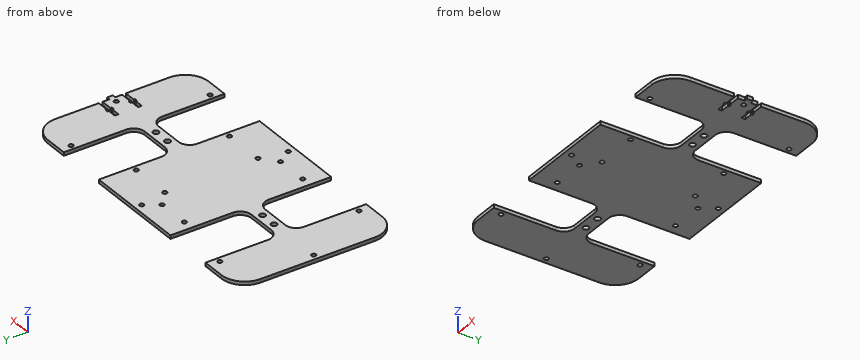
```python
from build123d import *

# Parameters (mm, degrees)
PAD_DEPTH       = 3
SKETCH004_R     = 2.5
POCKET_DEPTH    = 588.208656
SKETCH005_R     = 1.9
POCKET001_DEPTH = 588.208656
SKETCH014_R     = 1.9
POCKET008_DEPTH = 3.001
SKETCH025_R     = 1.9
POCKET016_DEPTH = 3.001
POCKET020_DEPTH = 588.208656
SKETCH032_W     = 3
SKETCH032_H     = 5
PAD007_DEPTH    = 3
SKETCH037_R     = 1.9
POCKET024_DEPTH = 593.505869


with BuildPart() as part:
    # Sketch → Pad (new body)
    with BuildSketch(Plane.XY):
        with BuildLine():
            Line((0, -69), (-45, -69))
            Line((-45, -69), (-45, -15.5))
            ThreePointArc((-45, -15.5), (-47.782486, -8.782486), (-54.5, -6))
            Line((-79.5, -6), (-54.5, -6))
            ThreePointArc((-79.5, -6), (-86.217514, -8.782486), (-89, -15.5))
            Line((-89, -69), (-89, -15.5))
            Line((-109.000046, -69), (-89, -69))
            ThreePointArc((-129, -48.999983), (-123.142158, -63.142113), (-109.000046, -69))
            Line((-129, 0), (-129, -48.999983))
            Line((-129, 0), (-129, 48.999983))
            ThreePointArc((-109.000046, 69), (-123.142158, 63.142113), (-129, 48.999983))
            Line((-109.000046, 69), (-89, 69))
            Line((-89, 69), (-89, 15.5))
            ThreePointArc((-89, 15.5), (-86.217514, 8.782485), (-79.5, 6))
            Line((-79.5, 6), (-54.5, 6))
            ThreePointArc((-54.5, 6), (-47.782485, 8.782485), (-45, 15.5))
            Line((-45, 69), (-45, 15.5))
            Line((0, 69), (-45, 69))
            Line((0, 69), (45, 69))
            Line((45, 69), (45, 15.5))
            ThreePointArc((45, 15.5), (47.782485, 8.782486), (54.499999, 6))
            Line((79.499999, 6), (54.499999, 6))
            ThreePointArc((79.499999, 6), (86.217514, 8.782486), (89, 15.5))
            Line((89, 69), (89, 15.5))
            Line((109.000054, 69), (89, 69))
            ThreePointArc((129, 48.999983), (123.142161, 63.142111), (109.000054, 69))
            Line((129, 0), (129, 48.999983))
            Line((129, 0), (129, -48.999983))
            ThreePointArc((109.000054, -69), (123.142161, -63.142111), (129, -48.999983))
            Line((109.000054, -69), (89, -69))
            Line((89, -69), (89, -15.5))
            ThreePointArc((89, -15.5), (86.217514, -8.782486), (79.5, -6))
            Line((79.5, -6), (54.5, -6))
            ThreePointArc((54.5, -6), (47.782486, -8.782486), (45, -15.5))
            Line((45, -69), (45, -15.5))
            Line((0, -69), (45, -69))
        make_face()
    extrude(amount=PAD_DEPTH)

    # Sketch004 (on Face30 of Pad) → Pocket (cut, through all)
    with BuildSketch(Plane.XY.offset(3)):
        with Locations((-74.25, 0)):
            Circle(SKETCH004_R)
        with Locations((-59.75, 0)):
            Circle(SKETCH004_R)
    pocket = extrude(amount=-POCKET_DEPTH, mode=Mode.SUBTRACT)

    # Mirrored: Pocket across Sketch004 V_Axis
    add(pocket.mirror(Plane(origin=(0, 0, 3), x_dir=(0, 0, 1), z_dir=(1, 0, 0))), mode=Mode.SUBTRACT)

    # Sketch005 (on Face30 of Clone) → Pocket001 (cut, through all)
    with BuildSketch(Plane.XY.offset(3)):
        with Locations((-124, 0)):
            Circle(SKETCH005_R)
        with Locations((-93.52, -59.69)):
            Circle(SKETCH005_R)
        with Locations((-93.52, 59.69)):
            Circle(SKETCH005_R)
    pocket001 = extrude(amount=-POCKET001_DEPTH, mode=Mode.SUBTRACT)

    # Mirrored006: Pocket001 across Sketch005 V_Axis
    add(pocket001.mirror(Plane(origin=(0, 0, 3), x_dir=(0, 0, 1), z_dir=(1, 0, 0))), mode=Mode.SUBTRACT)

    # Sketch014 (on Face5 of Mirrored006) → Pocket008 (cut, through all)
    with BuildSketch(Plane.XY.offset(3)):
        with Locations((-35.94, 50.8)):
            Circle(SKETCH014_R)
        with Locations((-8, 50.8)):
            Circle(SKETCH014_R)
        with Locations((-8, -50.8)):
            Circle(SKETCH014_R)
        with Locations((-35.94, -50.8)):
            Circle(SKETCH014_R)
    extrude(amount=-POCKET008_DEPTH, mode=Mode.SUBTRACT)

    # Sketch025 (on Face5 of Pocket008) → Pocket016 (cut, through all)
    with BuildSketch(Plane.XY.offset(3)):
        with Locations((40.5, -40)):
            Circle(SKETCH025_R)
        with Locations((4.5, 40)):
            Circle(SKETCH025_R)
        with Locations((4.5, -40)):
            Circle(SKETCH025_R)
        with Locations((40.5, 40)):
            Circle(SKETCH025_R)
    extrude(amount=-POCKET016_DEPTH, mode=Mode.SUBTRACT)

    # Sketch031 (on ShapeBinder) → Pocket020 (cut, through all)
    with BuildSketch(Plane.XY.offset(3)):
        Polygon((129, 8.4), (129, 11.6), (119, 11.6), (119, 12.75), (116.5, 12.75), (116.5, 11.6), (109, 11.6), (109, 8.4), (116.5, 8.4), (116.5, 7.25), (119, 7.25), (119, 8.4), align=None)
    pocket020 = extrude(amount=-POCKET020_DEPTH, mode=Mode.SUBTRACT)

    # Mirrored018: Pocket020 across Sketch031 H_Axis
    add(pocket020.mirror(Plane(origin=(0, 0, 3), x_dir=(0, 0, 1), z_dir=(0, 1, 0))), mode=Mode.SUBTRACT)

    # Sketch032 (on ShapeBinder) → Pad007 (join)
    with BuildSketch(Plane.XY.offset(3)):
        with Locations((130.5, 0)):
            Rectangle(SKETCH032_W, SKETCH032_H)
    extrude(amount=-PAD007_DEPTH)

    # Sketch037 (on Face80 of Pad007) → Pocket024 (cut, through all)
    with BuildSketch(Plane.XY.offset(3)):
        with Locations((0, 63)):
            Circle(SKETCH037_R)
    pocket024 = extrude(amount=-POCKET024_DEPTH, mode=Mode.SUBTRACT)

    # Mirrored020: Pocket024 across Sketch037 H_Axis
    add(pocket024.mirror(Plane(origin=(0, 0, 3), x_dir=(0, 0, 1), z_dir=(0, 1, 0))), mode=Mode.SUBTRACT)


solid = part.part
```
For this review, take the finished solid that the model builds, in its own axes (mm). Give positions to 0.01 mm unless a question says otherwise; leave off trailing zeros. Write each loop counter-clockwise with the first axis right and the second up, starting at its lowest first coordinate (ties: lowest second). Pieces come first, ordered by that corner, then holes.
Item 1: Insertion check: P1, Ø8, axis at x = 74.25, y = 0, coming from the -Z side; P2, Ø1.5, axis at x = 66, z = 1.5, coming from the +Y side; P3, Ø1.5, axis at y = -30.5, z = 1, coming from the +X side; P4, Ø0.8, axis at x = 118, z = 2, coming from the -Y side. Each pin has a flat end and moves straight along its axis. Give the tip position at first contact, or say it passes through.
Item 2: Wall thickness on probe 1 along X at (y, z) = (31.5, 0.2); probe 2 along Y at (x, z) = (-35.94, 1.25); probe 3 along Y at (x, z) = (-59.75, 1.2): over which ranges is each line inside the solid? List them lowest first.
Item 3: Take a section at B-B (x = 59.75). Give the boundary of the cut face in (y, z).
Item 4: Take a section at A-A (y = 35.5). Give the boundary of the cut face in (x, z), and give its area (3 significant figures).
Item 5: Take a section at C-C (z = 1.9). Give the number of separate pieces and of enclosed holes in the cut face, and give its area (3 significant figures).
Established:
1. P1: stops at z = 0
1. P2: stops at y = 6
1. P3: stops at x = 129
1. P4: stops at y = -67.06
2. probe 1: x = -129 to -89, -45 to 45, 89 to 129
2. probe 2: y = -69 to -52.7, -48.9 to 48.9, 52.7 to 69
2. probe 3: y = -6 to -2.5, 2.5 to 6
3. outline: (-6, 0) - (-2.5, 0) - (-2.5, 3) - (-6, 3) - close; (2.5, 0) - (6, 0) - (6, 3) - (2.5, 3) - close
4. outline: (-129, 0) - (-89, 0) - (-89, 3) - (-129, 3) - close; (-45, 0) - (45, 0) - (45, 3) - (-45, 3) - close; (89, 0) - (129, 0) - (129, 3) - (89, 3) - close
4. area: 510 mm2
5. separate pieces: 1
5. enclosed holes: 20
5. area: 23,900 mm2
